Autodesk Inventor part; units mm, degrees
ref_plane "YZ Plane" through (0, 0, 0) normal (1, 0, 0) x (0, 1, 0)
ref_plane "XZ Plane" through (0, 0, 0) normal (0, 1, 0) x (-1, 0, 0)
ref_plane "XY Plane" through (0, 0, 0) normal (0, 0, 1) x (1, 0, 0)
sketch "Sketch1" plane through (0, 0, 0) normal (0, 0, 1) x (1, 0, 0)
  circle A0 centre (0, 0) radius 3.5719
  dimension "d10" = 7.1437
extrude "Extrusion1" add sketch "Sketch1" along normal blind 45.2438
sketch "Sketch2" plane through (0, 0, 45.2438) normal (0, 0, 1) x (1, 0, 0)
  arc A0 (-1.7749, 1.5875) -> (1.7749, 1.5875) centre (0, 0) ccw
  line L0 (1.7749, 1.5875) -> (-1.7749, 1.5875)
  circle A1 centre (0, 0) radius 3.5719
  dimension "d2" = 4.7625
extrude "Extrusion2" cut sketch "Sketch2" against normal blind 17.4625
sketch "Sketch3" plane through (0, 0, 45.2438) normal (0, 0, 1) x (1, 0, 0)
  circle A0 centre (0, 0) radius 1.143
  dimension "d5" = 2.286
extrude "Extrusion3" cut sketch "Sketch3" against normal blind 3.175
chamfer "Chamfer1" distance 0.127 angle 45 5 edges at (0, -2.3813, 45.2438) (0, 1.5875, 45.2438) (-1.143, 0, 45.2438) (-3.5719, 0, 27.7813) (-3.5719, 0, 0)
properties part number "shaft" material "Brass, Soft Yellow"
Geometry check sheet. Reference: the model listing, model coordinates, mm. A direction names the side the tool comes from. Coordinates: 2 decimals unless noted, no trailing zeros. Write each loop counter-clockwise with the first axis right and the second up, starting at its lowest first coordinate (ties: lowest second). Pieces come first, ordered by that corner, then holes. Notation, with made-up numbers: (-10.5, 65) -> (12.5, 65) arc R27 cw to (12.5, 89) -> close; hole circle Ø3 at (68.5, 36.5). An arc over 180 degrees is marked (long way). One line per question, with ' | ' between items.
1. Cross-section at A-A on x = 0. Record the cut outline in (y, z), and give its area (3 significant figures).
Answers:
outline: (-3.57, 0.13) -> (-3.44, 0) -> (3.44, 0) -> (3.57, 0.13) -> (3.57, 27.65) -> (3.44, 27.78) -> (1.59, 27.78) -> (1.59, 45.12) -> (1.46, 45.24) -> (1.27, 45.24) -> (1.14, 45.12) -> (1.14, 42.07) -> (-1.14, 42.07) -> (-1.14, 45.12) -> (-1.27, 45.24) -> (-2.25, 45.24) -> (-2.38, 45.12) -> (-2.38, 27.78) -> (-3.44, 27.78) -> (-3.57, 27.65) -> close | area: 260 mm²
2. Draft check along X on faces 3 (the flat face through (0, 0, 42.069)), 4 (the flat face through (0, 1.588, 37)), 5 (the cylindrical face through (-0.248, -1.116, 43.614)), 6 (the cylindrical face through (-0.08, -2.38, 36.57)). Enter one of: +X half, -X half, draft (parallel to the pull), parting line (faces both ways), or undercut.
Answers:
face 3: undercut | face 4: draft | face 5: undercut | face 6: parting line
3. Cross-section at D-D on z = 14. Record the cut outline in (x, y), and give its area (3 significant figures).
Answers:
outline: circle Ø7.14 at (0, 0) | area: 40.1 mm²
4. Set-up check for faces 1 (the flat face through (0, 2, 27.781)), 2 (the flat face through (0, -2, 45.244)): record each of +Z, -Z, +X, -X, +Y, -Y from which the full face is reachable in a straight line by a thin tool's end or side.
Answers:
face 1: +Z | face 2: +Z, +X, -X, +Y, -Y
5. Cross-section at B-B on y = 0. Record the cut outline in (x, z).
Answers:
outline: (-3.57, 0.13) -> (-3.44, 0) -> (3.44, 0) -> (3.57, 0.13) -> (3.57, 27.65) -> (3.44, 27.78) -> (2.38, 27.78) -> (2.38, 45.12) -> (2.25, 45.24) -> (1.27, 45.24) -> (1.14, 45.12) -> (1.14, 42.07) -> (-1.14, 42.07) -> (-1.14, 45.12) -> (-1.27, 45.24) -> (-2.25, 45.24) -> (-2.38, 45.12) -> (-2.38, 27.78) -> (-3.44, 27.78) -> (-3.57, 27.65) -> close
6. Depth check by flat-ended pin: pin 1 Ø3 at (y, z) = (3, 36.5) entering from -X; pin 2 Ø2 at (x, z) = (2, 8.5) entering from +Y; pin 3 Ø1.8 at (x, z) = (-0.5, 40.5) entering from +Y. Enter the tip coordinate at first touch or a pass-through.
Answers:
pin 1: stops at x = -1.85 | pin 2: stops at y = 3.43 | pin 3: stops at y = 1.59
7. Cross-section at C-C on z = 39.5. Record the cut outline in (x, y).
Answers:
outline: (-1.77, 1.59) arc R2.38 ccw (long way) to (1.77, 1.59) -> close
8. Thickness scan on probe 1 along Y at (x, z) = (0, 44.2); probe 2 along Z at (x, y) = (0.25, -2.25); probe 3 along Z at (x, y) = (0, -2.5). Record the ranges inside material, lowest first. Write a range as from..to.
Answers:
probe 1: y = -2.38..-1.14, 1.14..1.59 | probe 2: z = 0..45.23 | probe 3: z = 0..27.78
